```python
from build123d import *

# Parameters (mm, degrees)
BOSS_EXTRUDE1_DEPTH             = 41.5
BOSS_EXTRUDE1_DEPTH_BACK        = 47
SKETCH2_W                       = 34
SKETCH2_H                       = 94
BOSS_EXTRUDE2_DEPTH             = 15
SKETCH3_W                       = 50
SKETCH3_H                       = 88.5
CUT_EXTRUDE1_DEPTH              = 1
ADVANCEDHOLE1_START             = 0.018666706
ADVANCEDHOLE1_DEPTH             = 12.837085488
ADVANCEDHOLE1_START_2           = -3.481333294
ADVANCEDHOLE1_2_OUTLINE_R       = 2.15
ADVANCEDHOLE1_2_DEPTH           = 3.5
ADVANCEDHOLE2_START             = -11.986045339
ADVANCEDHOLE2_DEPTH             = 11.967378633
ADVANCEDHOLE2_START_2           = -0.018666706
ADVANCEDHOLE2_2_OUTLINE_R       = 2.15
ADVANCEDHOLE2_2_DEPTH           = 3.5
FILLET1_R                       = 4
M4_TAPPED_HOLE1_D               = 3.3
M4_TAPPED_HOLE1_DEPTH           = 9.1
M4_TAPPED_HOLE1_TIP             = 0.991420021
M4_TAPPED_HOLE1_ON_FACE_2_D     = 3.3
M4_TAPPED_HOLE1_ON_FACE_2_DEPTH = 9.1
M4_TAPPED_HOLE1_ON_FACE_2_TIP   = 0.991420021
M4_TAPPED_HOLE1_ON_FACE_3_D     = 3.3
M4_TAPPED_HOLE1_ON_FACE_3_DEPTH = 9.1
M4_TAPPED_HOLE1_ON_FACE_3_TIP   = 0.991420021
M4_TAPPED_HOLE1_ON_FACE_4_D     = 3.3
M4_TAPPED_HOLE1_ON_FACE_4_DEPTH = 9.1
M4_TAPPED_HOLE1_ON_FACE_4_TIP   = 0.991420021
CHAMFER1_SIZE                   = 2
CHAMFER2_SIZE                   = 1
CHAMFER2_SIZE2                  = 1.732050808
CUT_EXTRUDE2_REACH              = 62.613


# Read off the part's stored shape, not the designer's step: AdvancedHole1, AdvancedHole2
with BuildPart() as part:
    # Sketch1 → Boss-Extrude1 (new, two sides: drawn at the far end of the back side and taken through both)
    with BuildSketch(Plane(origin=(0, 0, 0), x_dir=(1, 0, 0), z_dir=(0, 1, 0)).offset(-BOSS_EXTRUDE1_DEPTH_BACK)):
        Polygon((17, 0), (20, 0), (17.52689899, 15.335150469), (15.598536161, 17.633283798), (9.470180616, 12.49098292), (8, 2), (-8, 2), (-9.470180616, 12.49098292), (-15.598536161, 17.633283798), (-17.52689899, 15.335150469), (-20, 0), (-17, 0), align=None)
    extrude(amount=BOSS_EXTRUDE1_DEPTH + BOSS_EXTRUDE1_DEPTH_BACK)

    # Sketch2 → Boss-Extrude2 (add)
    with BuildSketch(Plane.XY):
        Rectangle(SKETCH2_W, SKETCH2_H)
    extrude(amount=BOSS_EXTRUDE2_DEPTH)

    # Sketch3 → Cut-Extrude1 (cut)
    with BuildSketch(Plane.XY):
        with Locations((-42, -2.75)):
            Rectangle(SKETCH3_W, SKETCH3_H)
    extrude(amount=-CUT_EXTRUDE1_DEPTH, mode=Mode.SUBTRACT)

    # AdvancedHole1 outline → AdvancedHole1 (cut)
    with BuildSketch(Plane(origin=(0, 0, 0), x_dir=(0.7660444431189763, 0, -0.6427876096865414), z_dir=(0.6427876096865414, 0, 0.7660444431189763)).offset(ADVANCEDHOLE1_START)):
        with BuildLine():
            Line((22.985109569, 33.983742651), (23.606222085, 35.5))
            Line((23.606222085, 35.5), (22.985109569, 37.016257349))
            ThreePointArc((22.985109569, 37.016257349), (15.283628291, 35.5), (22.985109569, 33.983742651))
        make_face()
        with BuildLine():
            Line((22.985109569, -37.016257349), (23.606222085, -35.5))
            Line((23.606222085, -35.5), (22.985109569, -33.983742651))
            ThreePointArc((22.985109569, -33.983742651), (15.283628291, -35.5), (22.985109569, -37.016257349))
        make_face()
        with BuildLine():
            ThreePointArc((22.985109569, 1.516257349), (15.283628291, 0), (22.985109569, -1.516257349))
            Line((22.985109569, -1.516257349), (23.606222085, 0))
            Line((23.606222085, 0), (22.985109569, 1.516257349))
        make_face()
    extrude(amount=ADVANCEDHOLE1_DEPTH, mode=Mode.SUBTRACT)

    # AdvancedHole1 2 outline → AdvancedHole1 2 (cut)
    with BuildSketch(Plane(origin=(0, 0, 0), x_dir=(0.7660444431189763, 0, -0.6427876096865414), z_dir=(0.6427876096865414, 0, 0.7660444431189763)).offset(ADVANCEDHOLE1_START_2)):
        with Locations((19.283628291, 0)):
            Circle(ADVANCEDHOLE1_2_OUTLINE_R)
        with Locations((19.283628291, -35.5)):
            Circle(ADVANCEDHOLE1_2_OUTLINE_R)
        with Locations((19.283628291, 35.5)):
            Circle(ADVANCEDHOLE1_2_OUTLINE_R)
    extrude(amount=ADVANCEDHOLE1_2_DEPTH, mode=Mode.SUBTRACT)

    # AdvancedHole2 outline → AdvancedHole2 (cut)
    with BuildSketch(Plane(origin=(0, 0, 0), x_dir=(0.7660444431189767, 0, 0.6427876096865409), z_dir=(0.6427876096865409, 0, -0.7660444431189768)).offset(ADVANCEDHOLE2_START)):
        with BuildLine():
            Line((-23.606222085, 35.5), (-22.985109569, 33.983742651))
            ThreePointArc((-22.985109569, 33.983742651), (-15.283628291, 35.5), (-22.985109569, 37.016257349))
            Line((-22.985109569, 37.016257349), (-23.606222085, 35.5))
        make_face()
        with BuildLine():
            Line((-22.985109569, 1.516257349), (-23.606222085, 0))
            Line((-23.606222085, 0), (-22.985109569, -1.516257349))
            ThreePointArc((-22.985109569, -1.516257349), (-15.283628291, 0), (-22.985109569, 1.516257349))
        make_face()
        with BuildLine():
            Line((-22.985109569, -33.983742651), (-23.606222085, -35.5))
            Line((-23.606222085, -35.5), (-22.985109569, -37.016257349))
            ThreePointArc((-22.985109569, -37.016257349), (-15.283628291, -35.5), (-22.985109569, -33.983742651))
        make_face()
    extrude(amount=ADVANCEDHOLE2_DEPTH, mode=Mode.SUBTRACT)

    # AdvancedHole2 2 outline → AdvancedHole2 2 (cut)
    with BuildSketch(Plane(origin=(0, 0, 0), x_dir=(0.7660444431189767, 0, 0.6427876096865409), z_dir=(0.6427876096865409, 0, -0.7660444431189768)).offset(ADVANCEDHOLE2_START_2)):
        with Locations((-19.283628291, 35.5)):
            Circle(ADVANCEDHOLE2_2_OUTLINE_R)
        with Locations((-19.283628291, 0)):
            Circle(ADVANCEDHOLE2_2_OUTLINE_R)
        with Locations((-19.283628291, -35.5)):
            Circle(ADVANCEDHOLE2_2_OUTLINE_R)
    extrude(amount=ADVANCEDHOLE2_2_DEPTH, mode=Mode.SUBTRACT)

    # Fillet1
    fillet1_edges = [part.edges().sort_by_distance(p)[0] for p in [
        (-8, -2.75, -2),
        (8, -2.75, -2),
    ]]
    fillet(fillet1_edges, radius=FILLET1_R)

    # M4 Tapped Hole1
    with Locations(Plane(origin=(0, -47, 7.5), x_dir=(0, 0, -1), z_dir=(0, -1, 0))):
        with Locations((0, 0)):
            Hole(M4_TAPPED_HOLE1_D / 2, depth=M4_TAPPED_HOLE1_DEPTH)
            with Locations((0, 0, -(M4_TAPPED_HOLE1_DEPTH + M4_TAPPED_HOLE1_TIP / 2))):  # 118° drill point
                Cone(0, M4_TAPPED_HOLE1_D / 2, M4_TAPPED_HOLE1_TIP, mode=Mode.SUBTRACT)

    # M4 Tapped Hole1 on face 2
    with Locations(Plane(origin=(17, 37, 7.5), x_dir=(0, 0, 1), z_dir=(1, 0, 0))):
        with Locations((0, 0), (0, 74), (0, 37)):
            Hole(M4_TAPPED_HOLE1_ON_FACE_2_D / 2, depth=M4_TAPPED_HOLE1_ON_FACE_2_DEPTH)
            with Locations((0, 0, -(M4_TAPPED_HOLE1_ON_FACE_2_DEPTH + M4_TAPPED_HOLE1_ON_FACE_2_TIP / 2))):  # 118° drill point
                Cone(0, M4_TAPPED_HOLE1_ON_FACE_2_D / 2, M4_TAPPED_HOLE1_ON_FACE_2_TIP, mode=Mode.SUBTRACT)

    # M4 Tapped Hole1 on face 3
    with Locations(Plane(origin=(-17, -37, 7.5), x_dir=(0, 0, -1), z_dir=(-1, 0, 0))):
        with Locations((0, 0), (0, -74), (0, -37)):
            Hole(M4_TAPPED_HOLE1_ON_FACE_3_D / 2, depth=M4_TAPPED_HOLE1_ON_FACE_3_DEPTH)
            with Locations((0, 0, -(M4_TAPPED_HOLE1_ON_FACE_3_DEPTH + M4_TAPPED_HOLE1_ON_FACE_3_TIP / 2))):  # 118° drill point
                Cone(0, M4_TAPPED_HOLE1_ON_FACE_3_D / 2, M4_TAPPED_HOLE1_ON_FACE_3_TIP, mode=Mode.SUBTRACT)

    # M4 Tapped Hole1 on face 4
    with Locations(Plane(origin=(0, 47, 7.5), x_dir=(0, 0, 1), z_dir=(0, 1, 0))):
        with Locations((0, 0)):
            Hole(M4_TAPPED_HOLE1_ON_FACE_4_D / 2, depth=M4_TAPPED_HOLE1_ON_FACE_4_DEPTH)
            with Locations((0, 0, -(M4_TAPPED_HOLE1_ON_FACE_4_DEPTH + M4_TAPPED_HOLE1_ON_FACE_4_TIP / 2))):  # 118° drill point
                Cone(0, M4_TAPPED_HOLE1_ON_FACE_4_D / 2, M4_TAPPED_HOLE1_ON_FACE_4_TIP, mode=Mode.SUBTRACT)

    # Chamfer1
    chamfer1_edges = [part.edges().sort_by_distance(p)[0] for p in [
        (17, -47, 7.5),
        (17, 47, 7.5),
        (-17, 47, 7.5),
        (-17, -47, 7),
    ]]
    chamfer(chamfer1_edges, length=CHAMFER1_SIZE)

    # Chamfer2
    chamfer2_edges = [part.edges().sort_by_distance(p)[0] for p in [
        (17, 0, 15),
        (0, -47, 15),
        (0, 47, 15),
        (-17, 0, 15),
        (-16, 46, 15),
        (16, 46, 15),
        (-16, -46, 15),
        (16, -46, 15),
    ]]
    chamfer2_side = [part.faces().sort_by_distance(p)[0] for p in [
        (0, 0, 15),
    ]]
    chamfer(chamfer2_edges, length=CHAMFER2_SIZE, length2=CHAMFER2_SIZE2, reference=chamfer2_side[0])

    # Sketch9 → Cut-Extrude2 (cut, up to next)
    with BuildSketch(Plane.XY.offset(15), mode=Mode.PRIVATE) as cut_extrude2_sk1:
        with BuildLine():
            Line((-6, 32), (-6, -32))
            ThreePointArc((-6, -32), (-4.828427125, -34.828427125), (-2, -36))
            Line((-2, -36), (2, -36))
            ThreePointArc((2, -36), (4.828427125, -34.828427125), (6, -32))
            Line((6, -32), (6, 32))
            ThreePointArc((6, 32), (4.828427125, 34.828427125), (2, 36))
            Line((2, 36), (-2, 36))
            ThreePointArc((-2, 36), (-4.828427125, 34.828427125), (-6, 32))
        make_face()
    cut_extrude2_tool1 = extrude(cut_extrude2_sk1.sketch, amount=-CUT_EXTRUDE2_REACH, mode=Mode.PRIVATE) & part.part
    add(cut_extrude2_tool1.solids().sort_by_distance((0, 0, 15))[0], mode=Mode.SUBTRACT)


solid = part.part
```
Check sheet for the modelled part. Datum: model origin and axes. Units: mm. A direction names the side the tool comes from. Round coordinates to 2 decimals unless told otherwise and drop trailing zeros. Order: outer loops, then holes, each group sorted by start corner. A loop starts at its lowest first (then second) coordinate and runs counter-clockwise, first axis right, second up. Notation, with made-up numbers: (80, 8) -> (137, 8) arc R27 ccw to (137, 24) -> close; hole circle Ø6 at (77.5, 16). An arc over 180 degrees is marked (long way). One line per item, written item: value. Start each with the question number.
Q1. Set-up check for faces 4 (the face through (0.07, -42.39, 5.85)), 5 (the face through (6, 0, 6)), 6 (the face through (12.39, -0.07, 9.15)): record each of +Z, -Z, +X, -X, +Y, -Y from which the full face is reachable in a straight line by a thin tool's end or side.
Q2. Mould release check, pull along Z, two halves, no side actions. Record for faces 1 (the face through (-4.797, 34.859, 6.479)), 2 (the face through (-14.77, -35.35, -6.18)), 3 (the face through (-19, -2, -1)): pulls with the +Z half, pulls with the -Z half, needs draft (parallel to the pull), parting line crosses it, or undercut.
Q3. Cross-section at A-A (z = 4.5). Record the boundary of the cut face in (x, y), and give its area (3 significant figures).
Q4. Thickness scan on line 1 (Y direction, x = 10.5, z = 7.5); line 2 (X direction, y = -11, z = 1); line 3 (Y direction, x = -0.5, z = 12.5). Record the ranges inside material, lowest first.
Q5. Gauge pin test, flat ends, axial feed: pin 1 Ø4.5 at (y, z) = (-37, 7.5) entering from +X; pin 2 Ø1 at (y, z) = (15, -12.5) entering from +X; pin 3 Ø5.5 at (x, z) = (0, 7.5) entering from +Y; pin 4 Ø4.5 at (y, z) = (-15, 5.5) entering from -X. Record the tip position at first contact, or that the pin passes through.
Completed:
1. face 4: -Y
1. face 5: +Z, -Z
1. face 6: +X
2. face 1: needs draft
2. face 2: undercut
2. face 3: pulls with the +Z half
3. outline: (-17, -45) -> (-15, -47) -> (15, -47) -> (17, -45) -> (17, 45) -> (15, 47) -> (-15, 47) -> (-17, 45) -> close; hole (-6, -32) arc R4 ccw to (-2, -36) -> (2, -36) arc R4 ccw to (6, -32) -> (6, 32) arc R4 ccw to (2, 36) -> (-2, 36) arc R4 ccw to (-6, 32) -> close
3. area: 2,340 mm²
4. line 1: y = -47 to -38.65, -35.35 to -1.65, 1.65 to 35.35, 38.65 to 47
4. line 2: x = -17 to -6, 6 to 17
4. line 3: y = -47 to -36, 36 to 47
5. pin 1: stops at x = 17
5. pin 2: stops at x = 18.06
5. pin 3: stops at y = 47
5. pin 4: stops at x = -17
